The model under review builds one solid part; all positions refer to its coordinate system, in mm. A direction names the side the tool comes from. Round coordinates to 2 decimals unless told otherwise and drop trailing zeros. Write each loop counter-clockwise with the first axis right and the second up, starting at its lowest first coordinate (ties: lowest second). Pieces come first, ordered by that corner, then holes. Notation, with made-up numbers: (-23, 81) - (33, 81) arc R20 ccw to (33, 116) - close; hole circle Ø8 at (-11.75, -18). An arc over 180 degrees is marked (long way). Write each question's results on one line, items separated by ' | '.
```python
from build123d import *

# Parameters (mm, degrees)
BOSS_EXTRUDE1_DEPTH      = 914.4
BOSS_EXTRUDE1_DEPTH_BACK = 914.4
SKETCH5_W                = 609.6
SKETCH5_H                = 38.1
CUT_EXTRUDE1_DEPTH       = 39.1


with BuildPart() as part:
    # Sketch4 → Boss-Extrude1 (new body, two sides)
    with BuildSketch(Plane(origin=(0, 0, 0), x_dir=(0, 0, -1), z_dir=(1, 0, 0))) as boss_extrude1_sk:
        with BuildLine():
            Line((19.05, -17.145), (19.05, 17.145))
            ThreePointArc((19.05, 17.145), (18.492038418, 18.492038418), (17.145, 19.05))
            Line((17.145, 19.05), (-17.145, 19.05))
            ThreePointArc((-17.145, 19.05), (-18.492038418, 18.492038418), (-19.05, 17.145))
            Line((-19.05, 17.145), (-19.05, -17.145))
            ThreePointArc((-19.05, -17.145), (-18.492038418, -18.492038418), (-17.145, -19.05))
            Line((-17.145, -19.05), (17.145, -19.05))
            ThreePointArc((17.145, -19.05), (18.492038418, -18.492038418), (19.05, -17.145))
        make_face()
        with BuildLine():
            Line((17.399, 15.6591), (17.399, -15.6591))
            ThreePointArc((17.399, -15.6591), (16.889395089, -16.889395089), (15.6591, -17.399))
            Line((15.6591, -17.399), (-15.6591, -17.399))
            ThreePointArc((-15.6591, -17.399), (-16.889395089, -16.889395089), (-17.399, -15.6591))
            Line((-17.399, -15.6591), (-17.399, 15.6591))
            ThreePointArc((-17.399, 15.6591), (-16.889395089, 16.889395089), (-15.6591, 17.399))
            Line((-15.6591, 17.399), (15.6591, 17.399))
            ThreePointArc((15.6591, 17.399), (16.889395089, 16.889395089), (17.399, 15.6591))
        make_face(mode=Mode.SUBTRACT)
    extrude(amount=BOSS_EXTRUDE1_DEPTH)
    extrude(boss_extrude1_sk.sketch, amount=-BOSS_EXTRUDE1_DEPTH_BACK)

    # Sketch5 → Cut-Extrude1 (cut, through all)
    with BuildSketch(Plane.XZ.offset(19.05)):
        with Locations((-609.6, 0)):
            Rectangle(SKETCH5_W, SKETCH5_H)
    extrude(amount=-CUT_EXTRUDE1_DEPTH, mode=Mode.SUBTRACT)


solid = part.part
```
Q1. Tool access review of faces 1 (the flat face through (313, -17.399, 0)), 2 (the flat face through (914.4, 0, 18)): name each direction out of +Z, -Z, +X, -X, +Y, -Y from which nothing blocks a thin tool from reaching the whole face with its end or side.
Evaluation:
face 1: +X, -X | face 2: +Z, -Z, +X, +Y, -Y
Q2. We need section A-A (x = 660.5). State the section outline as (y, z) points (3 decimals), plus the area to 3 significant figures.
Evaluation:
outline: (-19.05, -17.145) arc R1.905 ccw to (-17.145, -19.05) - (17.145, -19.05) arc R1.905 ccw to (19.05, -17.145) - (19.05, 17.145) arc R1.905 ccw to (17.145, 19.05) - (-17.145, 19.05) arc R1.905 ccw to (-19.05, 17.145) - close; hole (-17.399, -15.659) arc R1.74 ccw to (-15.659, -17.399) - (15.659, -17.399) arc R1.74 ccw to (17.399, -15.659) - (17.399, 15.659) arc R1.74 ccw to (15.659, 17.399) - (-15.659, 17.399) arc R1.74 ccw to (-17.399, 15.659) - close | area: 240 mm^2
Q3. The part is to be moulded in two halves that separate along Z. For faces 3 (the flat face through (313, 19.05, 0)), 4 (the flat face through (313, 0, -19.05)), 5 (the flat face through (313, 17.399, 0)), say which applies: released by +Z, released by -Z, zero draft, split by the parting line, or undercut.
Evaluation:
face 3: zero draft | face 4: released by -Z | face 5: undercut
Q4. For probe 1 along Y at (x, z) = (-153, 15.5); probe 2 along Z at (x, y) = (139, -16.5), list the stretches that pass through material, from the lowest coordinate up.
Evaluation:
probe 1: y = -19.05 to -17.4, 17.4 to 19.05 | probe 2: z = -19.05 to -17.18, 17.18 to 19.05
Q5. We need section B-B (z = -0.5). State the section outline as (x, y) points, plus the area to 3 significant figures.
Evaluation:
outline: (-304.8, -19.05) - (914.4, -19.05) - (914.4, -17.4) - (-304.8, -17.4) - close; (-304.8, 17.4) - (914.4, 17.4) - (914.4, 19.05) - (-304.8, 19.05) - close | area: 4,030 mm^2
